Geometry check sheet. Reference: the model listing, model coordinates, mm. A direction names the side the tool comes from. Round coordinates to 2 decimals unless told otherwise and drop trailing zeros. Order: outer loops, then holes, each group sorted by start corner. A loop starts at its lowest first (then second) coordinate and runs counter-clockwise, first axis right, second up. Notation, with made-up numbers: (-32.5, -24) - (15.5, -24) arc R28 ccw to (15.5, 11) - close; hole circle Ø7 at (48, 85.25). An arc over 180 degrees is marked (long way). Return JSON: item names as keys, results as strings. Group by question number.
Q1. Material ranges on line 1 along X through (y, z) = (15, 7.5); line 2 along Z through (x, y) = (-10.25, 4.5) (3 decimals); line 3 along Y through (x, z) = (-1, 12.75) (3 decimals), recorded low to high.
Q2. Sectioned sample at A-A, the plane z = 6. Record the cut outline in (x, y) (3 decimals).
Q3. Sectioned sample at B-B, the plane y = 12.75. Record the cut outline in (x, z) (3 decimals).
Q4. Gauge pin test, flat end, axial feed: pin 1 Ø4 at (x, y) = (-10, 0) entering from +Z (3 decimals). Record the tip position at first contact, or that the pin passes through.
Q5. Sectioned sample at C-C, the plane x = 2.5. Record the cut outline in (y, z) (3 decimals), then the cut area to 3 significant figures.
Q6. Draft check along X on faces 1 (the cylindrical face through (-8.5, 0.07, 1.61)), 2 (the flat face through (0, 18, 9)), 3 (the cylindrical face through (4.545, -4.646, 1.565)), 4 (the cylindrical face through (-5.074, 16.435, 15.671)). Enter one of: pulls with the +X half, pulls with the -X half, needs draft (parallel to the pull), parting line crosses it, or undercut.
Q7. Tool access check on faces 5 (the flat face through (-6.5, 16, 5)), 6 (the cylindrical face through (-0.575, 16.435, 12.561)), 7 (the flat face through (0, 14.825, 9)). Record the directions out of +Z, -Z, +X, -X, +Y, -Y that give a thin tool (end or side, any length) a straight path to the whole face; none if there is none.
```python
from build123d import *

# Parameters (mm, degrees)
SKETCH1_R               = 6.5
SKETCH1_R_2             = 1.5
BOSS_EXTRUDE1_DEPTH     = 3.175
SKETCH2_W               = 13
SKETCH2_H               = 3.175
BOSS_EXTRUDE2_DEPTH     = 14
SKETCH3_R               = 1.5
CUT_EXTRUDE1_DEPTH      = 18
FILLET1_R               = 5
BOSS_EXTRUDE3_START     = -3.175
BOSS_EXTRUDE3_OUTLINE_R = 1.5
BOSS_EXTRUDE3_DEPTH     = 3.175
FILLET3_R               = 1
CHAMFER1_SIZE           = 5


with BuildPart() as part:
    # Sketch1 → Boss-Extrude1 (new body)
    # profile 1 of 2: a face of its own
    with BuildSketch(Plane.XY):
        Circle(SKETCH1_R)
        Circle(SKETCH1_R_2, mode=Mode.SUBTRACT)
    # profile 2 of 2: a face of its own
    with BuildSketch(Plane.XY):
        with BuildLine():
            Line((-6.5, 18), (-6.5, 0))
            ThreePointArc((-6.5, 0), (0, 6.5), (6.5, 0))
            Line((6.5, 0), (6.5, 18))
            Line((6.5, 18), (-6.5, 18))
        make_face()
    extrude(amount=BOSS_EXTRUDE1_DEPTH)

    # Sketch2 → Boss-Extrude2 (add)
    with BuildSketch(Plane.XY.offset(3.175)):
        with Locations((0, 16.4125)):
            Rectangle(SKETCH2_W, SKETCH2_H)
    extrude(amount=BOSS_EXTRUDE2_DEPTH)

    # Sketch3 → Cut-Extrude1 (cut)
    with BuildSketch(Plane(origin=(0, 18, 0), x_dir=(1, 0, 0), z_dir=(0, 1, 0))):
        with Locations(Location((0, -11.175, 0), (0, 0, 270))):
            Circle(SKETCH3_R)
    extrude(amount=-CUT_EXTRUDE1_DEPTH, mode=Mode.SUBTRACT)

    # Fillet1
    fillet1_edges = [part.edges().sort_by_distance(p)[0] for p in [
        (-6.5, 16.4125, 17.175),
        (6.5, 16.4125, 17.175),
    ]]
    fillet(fillet1_edges, radius=FILLET1_R)

    # Boss-Extrude3: read off the stored shape, not the designer's step
    # Boss-Extrude3 outline → Boss-Extrude3 (add)
    with BuildSketch(Plane(origin=(0, 0, 0), x_dir=(-1, 0, 0), z_dir=(0, 0, -1)).offset(BOSS_EXTRUDE3_START)):
        with BuildLine():
            ThreePointArc((6.5, 0), (4.596194078, -4.596194078), (0, -6.5))
            Line((0, -6.5), (10, -6.5))
            ThreePointArc((10, -6.5), (16.239069091, 1.823188658), (6.5, 5.477225575))
            Line((6.5, 5.477225575), (6.5, 0))
        make_face()
        with Locations((10, 0)):
            Circle(BOSS_EXTRUDE3_OUTLINE_R, mode=Mode.SUBTRACT)
    extrude(amount=BOSS_EXTRUDE3_DEPTH)

    # Fillet3
    fillet3_edges = [part.edges().sort_by_distance(p)[0] for p in [
        (0, 14.825, 3.175),
        (0, 18, 0),
    ]]
    fillet(fillet3_edges, radius=FILLET3_R)

    # Chamfer1
    # the kernel refuses this chamfer: 5, 3.62027218 mm, written as the material it adds along each edge
    with BuildSketch(Plane(origin=(-6.5, 5.477225575, 3.175), x_dir=(0, 1, 0), z_dir=(0, 0, -1))) as chamfer1_piece_1:
        with BuildLine():
            Line((CHAMFER1_SIZE, 0), (1.003807775, -3.996192225))
            ThreePointArc((1.003807775, -3.996192225), (0.840081721, -1.969761939), (0, 0))
            Line((0, 0), (CHAMFER1_SIZE, 0))
        make_face()
    extrude(amount=3.175)


solid = part.part
```
Reply:
{
 "1": {"line 1": "-6.5 to 6.5", "line 2": "0 to 3.175", "line 3": "14.825 to 18"},
 "2": {"outline": "(-6.5, 14.825) - (6.5, 14.825) - (6.5, 18) - (-6.5, 18) - close"},
 "3": {"outline": "(-6.5, 0) - (6.5, 0) - (6.5, 3.175) - (-6.5, 3.175) - close"},
 "4": {"pin 1": "z = 3.175"},
 "5": {"outline": "(-6, 0) - (17, 0) arc R1 ccw to (18, 1) - (18, 17.074) - (14.825, 17.074) - (14.825, 4.175) arc R1 cw to (13.825, 3.175) - (-6, 3.175) - close", "area": "120 mm^2"},
 "6": {"face 1": "undercut", "face 2": "needs draft", "face 3": "pulls with the +X half", "face 4": "pulls with the -X half"},
 "7": {"face 5": "+Z, -Z, -X, +Y", "face 6": "+Y, -Y", "face 7": "+Z, +X, -X, -Y"}
}
